Check sheet for the modelled part. Datum: model origin and axes. Units: mm. Face numbers are marked on the shaded views. A direction names the side the tool comes from. Coordinates: 2 decimals unless noted, no trailing zeros. Order: outer loops, then holes, each group sorted by start corner. A loop starts at its lowest first (then second) coordinate and runs counter-clockwise, first axis right, second up.
from build123d import *

# Parameters (mm, degrees)
F2_R = 4.8284271247
F3_R = 4.99999
F4_R = 5
F5_R = 5
F6_R = 5
F7_R = 5


# Not quite as in the source:
# - a fillet or chamfer is up to 0.001 mm smaller than in the source, because OpenCascade refuses the exact size


with BuildPart() as f1:
    # F0 (on Front) → F1 (revolve)
    with BuildSketch(Plane.XZ):
        Polygon((0, 55.4385791123), (0, -7.8231290636), (15, -7.8231290636), (15, 3.1768709364), (10, 3.1768709364), (10, 23.6928891391), (5, 23.6928891391), (5, 55.4385791123), (10, 55.4385791123), (18, 67.4385791123), (9, 64.4385791123), (0, 72.1768709364), (0, 61.4385791123), align=None)
    revolve(axis=Axis((0, 0, 26.8077250243), (0, 0, 1)))

    # F2
    f2_edges = [f1.edges().sort_by_distance(p)[0] for p in [
        (-10, 0, 23.692889),
    ]]
    fillet(f2_edges, radius=F2_R)

    # F3 (radius 5 in the source; OpenCascade refuses exactly that, so slightly less here)
    f3_edges = [f1.edges().sort_by_distance(p)[0] for p in [
        (-15, 0, 3.176871),
    ]]
    fillet(f3_edges, radius=F3_R)

    # F4
    f4_edges = [f1.edges().sort_by_distance(p)[0] for p in [
        (-5, 0, 23.692889),
    ]]
    fillet(f4_edges, radius=F4_R)

    # F5
    f5_edges = [f1.edges().sort_by_distance(p)[0] for p in [
        (-10, 0, 55.438579),
    ]]
    fillet(f5_edges, radius=F5_R)

    # F6
    f6_edges = [f1.edges().sort_by_distance(p)[0] for p in [
        (-9, 0, 64.438579),
    ]]
    fillet(f6_edges, radius=F6_R)

    # F7
    f7_edges = [f1.edges().sort_by_distance(p)[0] for p in [
        (-5, 0, 55.438579),
    ]]
    fillet(f7_edges, radius=F7_R)


solid = f1.part
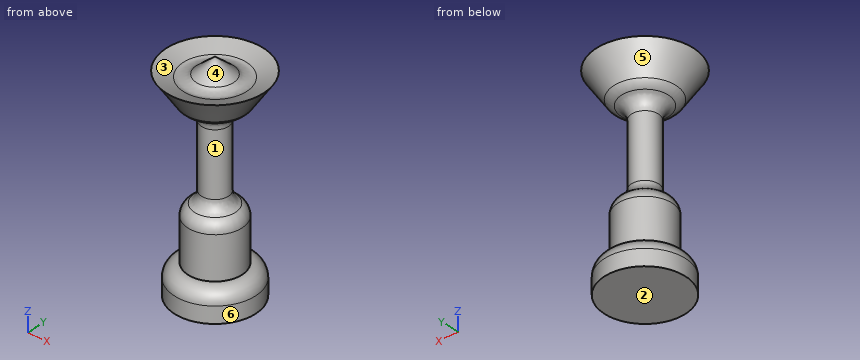
(1) Cross-section at B-B (z = 7). Enter the section's corners in (x, y), and give its area (3 significant figures).
Filled in:
outline: circle Ø20 at (0, 0)
area: 314 mm2
(2) Go/stop test with flat-tipped pins: P1, Ø6, axis at y = 7.5, z = 20, coming from the +X side; P2, Ø3, axis at x = -13, y = 12, coming from the +Z side; P3, Ø3, axis at x = -9.5, z = 25.5, coming from the -Y side; P4, Ø4, axis at y = 9.5, z = 22.5, coming from the +X side. Record where each tip stops, or that it passes through.
Filled in:
P1: stops at x = 8.87
P2: stops at z = 67.44
P3: passes through
P4: stops at x = 4.99
(3) Release check for a two-part mould opening along X. For the marked faces 1, 2, 3 and 4 record: +X half, -X half, draft (parallel to the pull), parting line (faces both ways), or undercut.
Filled in:
face 1: parting line
face 2: draft
face 3: undercut
face 4: undercut
(4) Cross-section at A-A (z = 36.5). Enter the section's corners in (x, y).
Filled in:
outline: circle Ø10 at (0, 0)
(5) Tool access check on the marked faces 5 and 6. Record the directions out of +Z, -Z, +X, -X, +Y, -Y that give a thin tool (end or side, any length) a straight path to the whole face; none if there is none.
Filled in:
face 5: none
face 6: -Z
(6) Thickness scan on probe 1 along Z at (x, y) = (7, -5); probe 2 along Z at (x, y) = (9, 5); probe 3 along Y at (x, z) = (-0.5, 11). Record the ranges inside material, lowest first.
Filled in:
probe 1: z = -7.82 to 22.26, 55.6 to 65.31
probe 2: z = -7.82 to 3.17, 56.42 to 65.08
probe 3: y = -9.99 to 9.99
